Input: part model. Units: mm. Frame: model coordinates. Round coordinates to 2 decimals unless told otherwise and drop trailing zeros. Loops run counter-clockwise (first coordinate to the right, second up) from the corner with the lowest first, then second, coordinate; pieces in that order, holes last. Notation, with made-up numbers: (47.25, 54) -> (63.25, 54) arc R25 ccw to (63.25, 84) -> close; hole circle Ø9 at (18.5, 79.25). An arc over 180 degrees is marked (long way). Answer in a Markdown table with one row per item. Add a question column.
Q1. Section A-A, the plane x = -65.5. Output: boundary loops of the cut face in (y, z).
Q2. Section C-C, the plane z = -76.5. Output: boundary loops of the cut face in (x, y).
Q3. Pin query (flat end, axial travel): pin 1 (12 mm diameter, centred on x = -92.5, z = -46.5, fed in from +Y); pin 2 (2.5 mm diameter, centred on y = 3.5, z = 115.5, fed in from +X); pin 3 (2 mm diameter, centred on x = -29, y = 1, fed in from +Z); pin 4 (1.5 mm diameter, centred on y = 2, z = 118.5, fed in from -X). Return the tip coordinate at first contact, or that it passes through.
Q4. Section D-D, the plane x = 1. Output: boundary loops of the cut face in (y, z), and give its area (3 significant figures).
Q5. Section B-B, the plane z = 24. Output: boundary loops of the cut face in (x, y) (3 decimals), and give its area (4 significant figures).
Q6. Ray query, L1, parallel to Z at x = -35, y = 3.2; L2, parallel to X at y = 1.7, z = -47.5; L3, parallel to X at y = 2.55, z = 81.5. Return the intervals inside material, ascending. Write a range as from..to.
```python
from build123d import *

# Parameters (mm, degrees)
SKETCH1_W               = 254
SKETCH1_H               = 254
PLATFORM_BASE_DEPTH     = 5.08
SKETCH9_W               = 25.4
SKETCH9_H               = 5.08
SKETCH9_W_2             = 19.05
CUT_EXTRUDE6_DEPTH      = 180.676950108
SKETCH3_R               = 1.75
CUT_EXTRUDE1_DEPTH      = 180.676950108
SKETCH4_W               = 63.5
SKETCH4_H               = 30.48
CUT_EXTRUDE2_DEPTH      = 180.676950108
CORNER_ROUNDING_R       = 25.4
SKETCH8_W               = 57.15
SKETCH8_H               = 57.15
CUT_EXTRUDE5_DEPTH      = 180.676950108
SKETCH10_W              = 50.8
SKETCH10_H              = 25.4
CUT_EXTRUDE7_DEPTH      = 180.676950108
SKETCH11_R              = 1.905
CUT_EXTRUDE8_DEPTH      = 180.676950108
SKETCH12_R              = 1.905
CUT_EXTRUDE9_DEPTH      = 180.676950108
SKETCH13_R              = 1.651
CUT_EXTRUDE10_DEPTH     = 180.676950108
MIRROR5_COPY_1_SKETCH_R = 1.651
MIRROR5_COPY_1_DEPTH    = 180.676950108
MIRROR7_COPY_1_SKETCH_W = 50.8
MIRROR7_COPY_1_SKETCH_H = 25.4
MIRROR7_COPY_1_DEPTH    = 180.676950108


with BuildPart() as part:
    # Sketch1 → Platform-Base (new body)
    with BuildSketch(Plane(origin=(0, 0, 0), x_dir=(1, 0, 0), z_dir=(0, 1, 0))):
        Rectangle(SKETCH1_W, SKETCH1_H)
    extrude(amount=PLATFORM_BASE_DEPTH)

    # Sketch9 → Cut-Extrude6 (cut, through all)
    with BuildSketch(Plane(origin=(0, 5.08, 0), x_dir=(1, 0, 0), z_dir=(0, 1, 0))):
        with Locations((-72.39, -114.3)):
            Rectangle(SKETCH9_W, SKETCH9_H)
        with Locations((72.39, -114.3)):
            Rectangle(SKETCH9_W, SKETCH9_H)
        with Locations((72.39, 114.3)):
            Rectangle(SKETCH9_W, SKETCH9_H)
        with Locations((-72.39, 114.3)):
            Rectangle(SKETCH9_W, SKETCH9_H)
        with Locations((72.39, -48.26)):
            Rectangle(SKETCH9_W, SKETCH9_H)
        with Locations((72.39, 48.26)):
            Rectangle(SKETCH9_W, SKETCH9_H)
        with Locations((-32.385, 48.26)):
            Rectangle(SKETCH9_W_2, SKETCH9_H)
        with Locations((-100.965, 48.26)):
            Rectangle(SKETCH9_W_2, SKETCH9_H)
        with Locations((-32.385, -48.26)):
            Rectangle(SKETCH9_W_2, SKETCH9_H)
        with Locations((-100.970875941, -48.26)):
            Rectangle(SKETCH9_W_2, SKETCH9_H)
    extrude(amount=-CUT_EXTRUDE6_DEPTH, mode=Mode.SUBTRACT)

    # Sketch3 → Cut-Extrude1 (cut, through all)
    with BuildSketch(Plane(origin=(0, 5.08, 0), x_dir=(1, 0, 0), z_dir=(0, 1, 0))):
        with Locations(Location((15, -64.2, 0), (0, 0, 270))):
            Circle(SKETCH3_R)
        with Locations(Location((15, -88.2, 0), (0, 0, 270))):
            Circle(SKETCH3_R)
        with Locations(Location((-15, -88.2, 0), (0, 0, 270))):
            Circle(SKETCH3_R)
        with Locations(Location((-15, -64.2, 0), (0, 0, 270))):
            Circle(SKETCH3_R)
    cut_extrude1 = extrude(amount=-CUT_EXTRUDE1_DEPTH, mode=Mode.SUBTRACT)

    # Mirror2: Cut-Extrude1 across plane
    add(cut_extrude1.mirror(Plane.XY), mode=Mode.SUBTRACT)

    # Sketch4 → Cut-Extrude2 (cut, through all)
    with BuildSketch(Plane(origin=(0, 5.08, 0), x_dir=(1, 0, 0), z_dir=(0, 1, 0))):
        with Locations((0, -111.76)):
            Rectangle(SKETCH4_W, SKETCH4_H)
    cut_extrude2 = extrude(amount=-CUT_EXTRUDE2_DEPTH, mode=Mode.SUBTRACT)

    # Mirror3: Cut-Extrude2 across plane
    add(cut_extrude2.mirror(Plane.XY), mode=Mode.SUBTRACT)

    # Corner-Rounding
    corner_rounding_edges = [part.edges().sort_by_distance(p)[0] for p in [
        (127, 2.54, 127),
        (-127, 2.54, 127),
        (-127, 2.54, -127),
        (127, 2.54, -127),
    ]]
    fillet(corner_rounding_edges, radius=CORNER_ROUNDING_R)

    # Sketch8 → Cut-Extrude5 (cut, through all)
    with BuildSketch(Plane(origin=(0, 5.08, 0), x_dir=(1, 0, 0), z_dir=(0, 1, 0))):
        with Locations((69.85, 0)):
            Rectangle(SKETCH8_W, SKETCH8_H)
    extrude(amount=-CUT_EXTRUDE5_DEPTH, mode=Mode.SUBTRACT)

    # Sketch10 → Cut-Extrude7 (cut, through all)
    with BuildSketch(Plane(origin=(0, 5.08, 0), x_dir=(1, 0, 0), z_dir=(0, 1, 0))):
        with Locations((-57.15, -76.2)):
            Rectangle(SKETCH10_W, SKETCH10_H)
    cut_extrude7 = extrude(amount=-CUT_EXTRUDE7_DEPTH, mode=Mode.SUBTRACT)

    # Sketch11 → Cut-Extrude8 (cut, through all)
    with BuildSketch(Plane(origin=(0, 5.08, 0), x_dir=(1, 0, 0), z_dir=(0, 1, 0))):
        with Locations(Location((-15.24, -18.415, 0), (0, 0, 270))):
            Circle(SKETCH11_R)
        with Locations(Location((-15.24, 18.415, 0), (0, 0, 270))):
            Circle(SKETCH11_R)
        with Locations(Location((21.59, 18.415, 0), (0, 0, 270))):
            Circle(SKETCH11_R)
        with Locations(Location((21.59, -18.415, 0), (0, 0, 270))):
            Circle(SKETCH11_R)
    extrude(amount=-CUT_EXTRUDE8_DEPTH, mode=Mode.SUBTRACT)

    # Sketch12 → Cut-Extrude9 (cut, through all)
    with BuildSketch(Plane(origin=(0, 5.08, 0), x_dir=(1, 0, 0), z_dir=(0, 1, 0))):
        with Locations(Location((30.927856532, -35.704925997, 0), (0, 0, 270))):
            Circle(SKETCH12_R)
        with Locations(Location((-37.144143468, -35.704925997, 0), (0, 0, 270))):
            Circle(SKETCH12_R)
        with Locations(Location((26.101856532, 36.778592543, 0), (0, 0, 270))):
            Circle(SKETCH12_R)
        with Locations(Location((-30.032143468, 37.193074003, 0), (0, 0, 270))):
            Circle(SKETCH12_R)
    extrude(amount=-CUT_EXTRUDE9_DEPTH, mode=Mode.SUBTRACT)

    # Sketch13 → Cut-Extrude10 (cut, through all)
    with BuildSketch(Plane(origin=(0, 5.08, 0), x_dir=(1, 0, 0), z_dir=(0, 1, 0))):
        with Locations(Location((-86.36, -101.6, 0), (0, 0, 270))):
            Circle(SKETCH13_R)
        with Locations(Location((-122.36, -101.6, 0), (0, 0, 270))):
            Circle(SKETCH13_R)
        with Locations(Location((-122.36, -85.6, 0), (0, 0, 270))):
            Circle(SKETCH13_R)
        with Locations(Location((-86.36, -85.6, 0), (0, 0, 270))):
            Circle(SKETCH13_R)
    cut_extrude10 = extrude(amount=-CUT_EXTRUDE10_DEPTH, mode=Mode.SUBTRACT)

    # Mirror4: Cut-Extrude10 across plane
    add(cut_extrude10.mirror(Plane.XY), mode=Mode.SUBTRACT)

    # Mirror5: Cut-Extrude10 across plane
    add(cut_extrude10.mirror(Plane(origin=(0, 0, 0), x_dir=(0, 0, 1), z_dir=(1, 0, 0))), mode=Mode.SUBTRACT)

    # Mirror5 copy 1 sketch → Mirror5 copy 1 (cut, through all)
    with BuildSketch(Plane(origin=(0, 5.08, 0), x_dir=(-1, 0, 0), z_dir=(0, 1, 0))):
        with Locations(Location((-86.36, -101.6, 0), (0, 0, 270))):
            Circle(MIRROR5_COPY_1_SKETCH_R)
        with Locations(Location((-122.36, -101.6, 0), (0, 0, 270))):
            Circle(MIRROR5_COPY_1_SKETCH_R)
        with Locations(Location((-122.36, -85.6, 0), (0, 0, 270))):
            Circle(MIRROR5_COPY_1_SKETCH_R)
        with Locations(Location((-86.36, -85.6, 0), (0, 0, 270))):
            Circle(MIRROR5_COPY_1_SKETCH_R)
    extrude(amount=-MIRROR5_COPY_1_DEPTH, mode=Mode.SUBTRACT)

    # Mirror6: Cut-Extrude7 across plane
    add(cut_extrude7.mirror(Plane(origin=(0, 0, 0), x_dir=(0, 0, 1), z_dir=(1, 0, 0))), mode=Mode.SUBTRACT)

    # Mirror7: Cut-Extrude7 across plane
    add(cut_extrude7.mirror(Plane.XY), mode=Mode.SUBTRACT)

    # Mirror7 copy 1 sketch → Mirror7 copy 1 (cut, through all)
    with BuildSketch(Plane(origin=(0, 5.08, 0), x_dir=(-1, 0, 0), z_dir=(0, 1, 0))):
        with Locations((-57.15, -76.2)):
            Rectangle(MIRROR7_COPY_1_SKETCH_W, MIRROR7_COPY_1_SKETCH_H)
    extrude(amount=-MIRROR7_COPY_1_DEPTH, mode=Mode.SUBTRACT)


solid = part.part
```
Answer block:
| question | item | result |
|---|---|---|
| 1 | outline | (0, -127) -> (5.08, -127) -> (5.08, -116.84) -> (0, -116.84) -> close; (0, -111.76) -> (5.08, -111.76) -> (5.08, -88.9) -> (0, -88.9) -> close; (0, -63.5) -> (5.08, -63.5) -> (5.08, 63.5) -> (0, 63.5) -> close; (0, 88.9) -> (5.08, 88.9) -> (5.08, 111.76) -> (0, 111.76) -> close; (0, 116.84) -> (5.08, 116.84) -> (5.08, 127) -> (0, 127) -> close |
| 2 | outline | (-127, 0) -> (-82.55, 0) -> (-82.55, 5.08) -> (-127, 5.08) -> close; (-31.75, 0) -> (31.75, 0) -> (31.75, 5.08) -> (-31.75, 5.08) -> close; (82.55, 0) -> (127, 0) -> (127, 5.08) -> (82.55, 5.08) -> close |
| 3 | pin 1 | y = 5.08 |
| 3 | pin 2 | x = 123.63 |
| 3 | pin 3 | z = 96.52 |
| 3 | pin 4 | x = -121.2 |
| 4 | outline | (0, -96.52) -> (5.08, -96.52) -> (5.08, 96.52) -> (0, 96.52) -> close |
| 4 | area | 981 mm^2 |
| 5 | outline | (-127, 0) -> (41.275, 0) -> (41.275, 5.08) -> (-127, 5.08) -> close; (98.425, 0) -> (127, 0) -> (127, 5.08) -> (98.425, 5.08) -> close |
| 5 | area | 1,000 mm^2 |
| 6 | L1 | -127..-88.9, -63.5..-50.8, -45.72..45.72, 50.8..63.5, 88.9..127 |
| 6 | L2 | -127..-110.49, -91.44..-41.91, -22.86..59.69, 85.09..127 |
| 6 | L3 | -127..-82.55, -31.75..31.75, 82.55..127 |
